For this review, take the finished solid that the model builds, in its own axes (mm). Face numbers are marked on the shaded views. A direction names the side the tool comes from. Give positions to 0.01 mm unless a question says otherwise; leave off trailing zeros. Write each loop counter-clockwise with the first axis right and the second up, starting at its lowest first coordinate (ties: lowest second). Pieces come first, ordered by that corner, then holes.
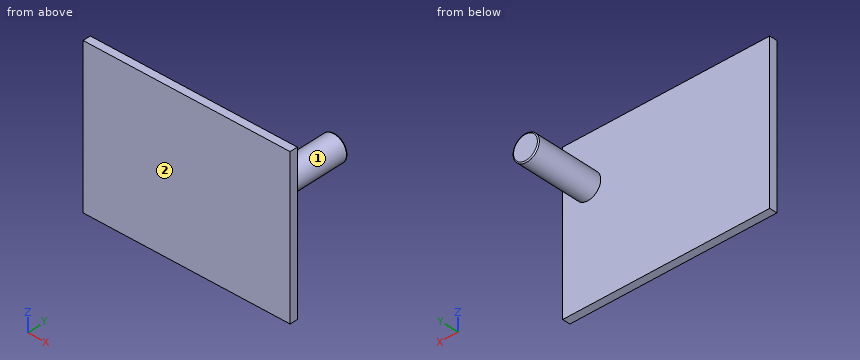
Autodesk Inventor part; units mm, degrees
ref_plane "YZ Plane" through (0, 0, 0) normal (1, 0, 0) x (0, 1, 0)
ref_plane "XZ Plane" through (0, 0, 0) normal (0, 1, 0) x (-1, 0, 0)
ref_plane "XY Plane" through (0, 0, 0) normal (0, 0, 1) x (1, 0, 0)
sketch "Sketch1" plane through (0, 0, 0) normal (0, 1, 0) x (-1, 0, 0)
  line L0 (0, 0) -> (40, 0)
  line L1 (40, 0) -> (40, -30)
  line L2 (40, -30) -> (0, -30)
  line L3 (0, -30) -> (0, 0)
  dimension "d0" = 40
  dimension "d1" = 30
extrude "Extrusion1" add sketch "Sketch1" along normal blind 1.5
sketch "Sketch2" plane through (0, 1.5, 0) normal (0, 1, 0) x (1, 0, 0)
  circle A0 centre (-4.8436, 9.1845) radius 2.5
  point P0 (0, 0)
  dimension "d4" = 5
extrude "Extrusion2" add sketch "Sketch2" along normal blind 13
fillet "Fillet1" radius 0.2 1 edges at (-7.3436, 14.5, -9.1845)
properties part number "Circuit_Board"
(1) We need section C-C (y = 7). Write out the cut boundary in (x, z), and give its area (3 significant figures).
(2) Clearance check with flat-ended pins moving along their axes: pin 1 Ø6 at (y, z) = (7, -6) entering from +X; pin 2 Ø3 at (x, z) = (-23, -19.5) entering from +Y; pin 3 Ø6 at (y, z) = (6, -17) entering from -X; pin 4 Ø8 at (y, z) = (8.5, -12.5) entering from +X. State where each tip first meets the part, or that it passes through.
(3) Tool access review of the marked faces 1 and 2: name each direction out of +Z, -Z, +X, -X, +Y, -Y from which nothing blocks a thin tool from reaching the whole face with its end or side.
(4) We need section A-A (z = -17). Write out the cut boundary in (x, y).
(5) For L1, parallel to Y at x = -22, z = -17.25; L2, parallel to Z at x = -5.5, y = 8; L3, parallel to X at y = 2.5, z = -9.5, list the stretches that pass through material, from the lowest coordinate up.
(6) We need section B-B (x = -10). Write out the cut boundary in (y, z).
The answers:
1. outline: circle Ø5 at (-4.84, -9.18)
1. area: 19.6 mm2
2. pin 1: stops at x = -2.35
2. pin 2: stops at y = 1.5
2. pin 3: passes through
2. pin 4: stops at x = -2.34
3. face 1: +Y
3. face 2: +Z, -Z, +X, -X, -Y
4. outline: (-40, 0) - (0, 0) - (0, 1.5) - (-40, 1.5) - close
5. L1: y = 0 to 1.5
5. L2: z = -11.6 to -6.77
5. L3: x = -7.32 to -2.36
6. outline: (0, -30) - (1.5, -30) - (1.5, 0) - (0, 0) - close
